Here's how the part is built. I have some questions about the finished solid (model axes, mm). Round coordinates to 2 decimals unless told otherwise and drop trailing zeros. Order: outer loops, then holes, each group sorted by start corner. A loop starts at its lowest first (then second) coordinate and runs counter-clockwise, first axis right, second up. Notation, with made-up numbers: M 67.5,-19.5 L 77.5,-19.5 A21 cw 77.5,-4.5 Z; hole C -6,-36 d8. An arc over 180 degrees is marked long. Write item = value, one per line. Start each with the question number.
Item 1: I want a section at C-C, the plane y = -47.5. List the corners of the cut face in (x, z) for me.
Item 2: I want a section at A-A, the plane y = 49.5. List the corners of the cut face in (x, z) for me.
Item 3: I'm going to push flat-ended pins straight in: P1, Ø4, axis at x = 30, y = 48, coming from the -Z side; P2, Ø9, axis at x = 19.05, y = -47.5, coming from the +Z side; P3, Ø2.5, axis at y = 0, z = 3, coming from the -X side; P4, Ø1.6, axis at y = -58, z = 2.5, coming from the +X side. Where does each tip first touch, or does it pass through?
Item 4: Please list where these lines run through material, in increasing order: L1, parallel to Y at x = 29.95, z = 0.7; L2, parallel to Y at x = -13.5, z = 4.75; L3, parallel to Y at x = -29, z = 6.25.
Item 5: I want a section at B-B, the plane x = 19.05. List the corners of the cut face in (y, z) for me, plus the area to 3 significant figures.
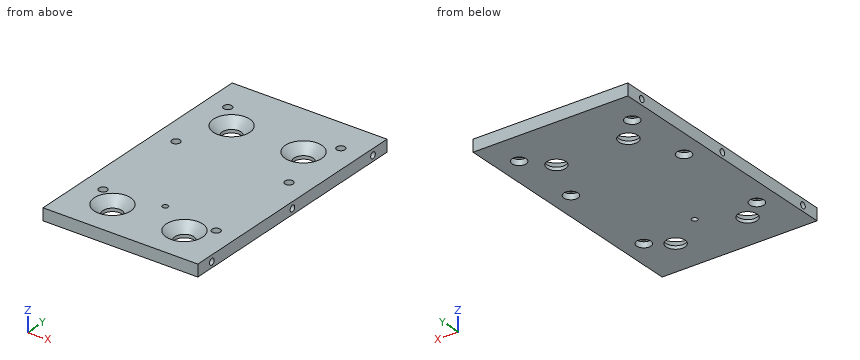
```python
from build123d import *

# Parameters (mm, degrees)
SKETCH1_W                                      = 82
SKETCH1_H                                      = 135
BOSS_EXTRUDE1_DEPTH                            = 6.35
CSK_FOR_M8_FLAT_HEAD_MACHINE_SCREW1_AT_2_COUNT = 2
CSK_FOR_M8_FLAT_HEAD_MACHINE_SCREW1_AT_2_PITCH = 38.1
CSK_FOR_M8_FLAT_HEAD_MACHINE_SCREW1_AT_3_COUNT = 2
CSK_FOR_M8_FLAT_HEAD_MACHINE_SCREW1_AT_3_PITCH = 85
CSK_FOR_M8_FLAT_HEAD_MACHINE_SCREW1_AT_4_COUNT = 2
CSK_FOR_M8_FLAT_HEAD_MACHINE_SCREW1_AT_4_PITCH = 93.148322583
SKETCH9_R                                      = 1.5
CUT_EXTRUDE2_DEPTH                             = 80.231133401
HOLE1_D                                        = 4.4
HOLE1_CBORE_D                                  = 7.5
HOLE1_CBORE_DEPTH                              = 3
SKETCH14_R                                     = 1.65
CUT_EXTRUDE4_DEPTH                             = 15


with BuildPart() as part:
    # Sketch1 → Boss-Extrude1 (new body)
    with BuildSketch(Plane.XY):
        Rectangle(SKETCH1_W, SKETCH1_H)
    extrude(amount=BOSS_EXTRUDE1_DEPTH)

    # Sketch4 → CSK for M8 Flat Head Machine Screw1 (revolve, cut)
    with BuildSketch(Plane(origin=(-19.05, 37.5, 6.35), x_dir=(0, -1, 0), z_dir=(1, 0, 0))):
        Polygon((0, 0), (0, 6.35), (5, 6.35), (5, 4.65), (9.65, 0), align=None)
    csk_for_m8_flat_head_machine_screw1 = revolve(axis=Axis((-19.05, 37.5, 12.7), (0, 0, -1)), mode=Mode.SUBTRACT)

    # CSK for M8 Flat Head Machine Screw1 at 2: CSK for M8 Flat Head Machine Screw1 ×2
    with Locations(*[(i * CSK_FOR_M8_FLAT_HEAD_MACHINE_SCREW1_AT_2_PITCH, 0, 0) for i in range(1, CSK_FOR_M8_FLAT_HEAD_MACHINE_SCREW1_AT_2_COUNT)]):
        add(csk_for_m8_flat_head_machine_screw1, mode=Mode.SUBTRACT)

    # CSK for M8 Flat Head Machine Screw1 at 3: CSK for M8 Flat Head Machine Screw1 ×2
    with Locations(*[(0, -i * CSK_FOR_M8_FLAT_HEAD_MACHINE_SCREW1_AT_3_PITCH, 0) for i in range(1, CSK_FOR_M8_FLAT_HEAD_MACHINE_SCREW1_AT_3_COUNT)]):
        add(csk_for_m8_flat_head_machine_screw1, mode=Mode.SUBTRACT)

    # CSK for M8 Flat Head Machine Screw1 at 4: CSK for M8 Flat Head Machine Screw1 ×2
    with Locations(*[Vector(0.4090250789659619, -0.9125231420500461, 0) * (i * CSK_FOR_M8_FLAT_HEAD_MACHINE_SCREW1_AT_4_PITCH) for i in range(1, CSK_FOR_M8_FLAT_HEAD_MACHINE_SCREW1_AT_4_COUNT)]):
        add(csk_for_m8_flat_head_machine_screw1, mode=Mode.SUBTRACT)

    # Sketch9 → Cut-Extrude2 (cut, through all)
    with BuildSketch(Plane(origin=(0, 0, 0), x_dir=(-1, 0, 0), z_dir=(0, 0, -1))):
        with Locations((0, -35.5)):
            Circle(SKETCH9_R)
    extrude(amount=-CUT_EXTRUDE2_DEPTH, mode=Mode.SUBTRACT)

    # Hole1 (through all)
    with Locations(Plane(origin=(0, 0, 0), x_dir=(-1, 0, 0), z_dir=(0, 0, -1))):
        with Locations((-29.95, -39.5), (-29.95, 12.5), (-29.95, 49.5), (29.95, 49.5), (29.95, 12.5), (29.95, -39.5)):
            CounterBoreHole(HOLE1_D / 2, HOLE1_CBORE_D / 2, HOLE1_CBORE_DEPTH)

    # Sketch14 → Cut-Extrude4 (cut)
    with BuildSketch(Plane(origin=(41, 0, 0), x_dir=(0, 0, -1), z_dir=(1, 0, 0))):
        with Locations(Location((-3, 57.5, 0), (0, 0, 90))):
            Circle(SKETCH14_R)
        with Locations(Location((-3, 0, 0), (0, 0, 90))):
            Circle(SKETCH14_R)
        with Locations(Location((-3, -57.5, 0), (0, 0, 90))):
            Circle(SKETCH14_R)
    cut_extrude4 = extrude(amount=-CUT_EXTRUDE4_DEPTH, mode=Mode.SUBTRACT)

    # Mirror1: Cut-Extrude4 across plane
    add(cut_extrude4.mirror(Plane(origin=(0, 0, 0), x_dir=(0, 0, 1), z_dir=(1, 0, 0))), mode=Mode.SUBTRACT)


solid = part.part
```
Filled in:
q1.outline = M -41,0 L -24.05,0 L -24.05,1.7 L -28.7,6.35 L -41,6.35 Z; M -14.05,0 L 14.05,0 L 14.05,1.7 L 9.4,6.35 L -9.4,6.35 L -14.05,1.7 Z; M 24.05,0 L 41,0 L 41,6.35 L 28.7,6.35 L 24.05,1.7 Z
q2.outline = M -41,0 L -33.7,0 L -33.7,3 L -32.15,3 L -32.15,6.35 L -41,6.35 Z; M -27.75,3 L -26.2,3 L -26.2,0 L 26.2,0 L 26.2,3 L 27.75,3 L 27.75,6.35 L -27.75,6.35 Z; M 32.15,3 L 33.7,3 L 33.7,0 L 41,0 L 41,6.35 L 32.15,6.35 Z
q3.P1 = 3
q3.P2 = through
q3.P3 = -26
q3.P4 = 26
q4.L1 = -67.5 to -43.25, -35.75 to 8.75, 16.25 to 45.75, 53.25 to 67.5
q4.L2 = -67.5 to -53.33, -41.67 to 31.67, 43.33 to 67.5
q4.L3 = -67.5 to -41.48, -37.52 to 10.52, 14.48 to 47.52, 51.48 to 67.5
q5.outline = M -67.5,0 L -52.5,0 L -52.5,1.7 L -57.15,6.35 L -67.5,6.35 Z; M -42.5,0 L 32.5,0 L 32.5,1.7 L 27.85,6.35 L -37.85,6.35 L -42.5,1.7 Z; M 42.5,0 L 67.5,0 L 67.5,6.35 L 47.15,6.35 L 42.5,1.7 Z
q5.area = 687 mm^2
